For this review, use the dimensioned drawing (mm, ordinates from the lowest corner) and the shaded views. Round coordinates to 2 decimals unless told otherwise and drop trailing zeros. Loops run counter-clockwise (first coordinate to the right, second up) from the corner with the lowest first, then second, coordinate; pieces in that order, holes last.
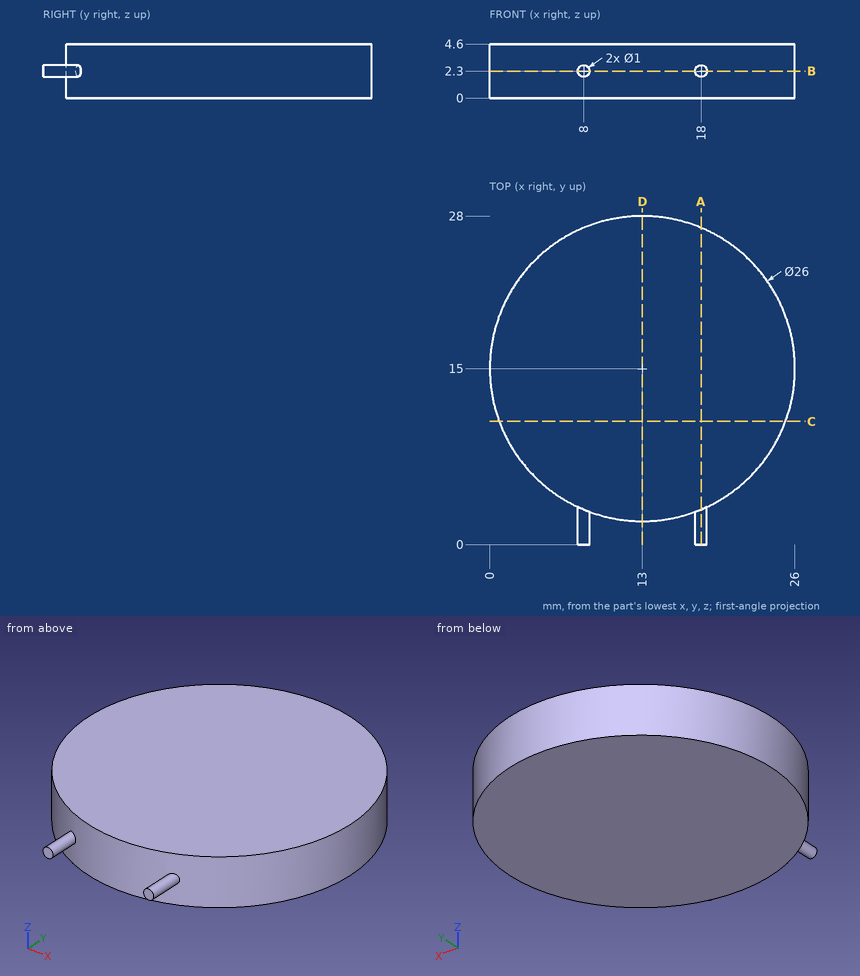
(1) For L1, parallel to Y at x = 2.25, z = 3.25; L2, parallel to Y at x = 15.5, z = 2.3; L3, parallel to X at y = 9.25, z = 2.4, list the stretches that pass through material, from the lowest coordinate up.
(2) Add section A-A (x = 18). Give the boundary of the cut face in (y, z).
(3) Add section D-D (x = 13). Give the boundary of the cut face in (y, z).
(4) Add section B-B (z = 2.3). Give the boundary of the cut face in (x, y).
(5) Add section C-C (y = 10.5). Give the boundary of the cut face in (x, z), plus the area to 3 significant figures.
Outcome:
1. L1: y = 7.69 to 22.31
1. L2: y = 2.24 to 27.76
1. L3: x = 1.34 to 24.66
2. outline: (0, 1.8) - (3, 1.8) - (3, 0) - (27, 0) - (27, 4.6) - (3, 4.6) - (3, 2.8) - (0, 2.8) - close
3. outline: (2, 0) - (28, 0) - (28, 4.6) - (2, 4.6) - close
4. outline: (7.5, 0) - (8.5, 0) - (8.5, 2.8) arc R13 ccw to (17.5, 2.8) - (17.5, 0) - (18.5, 0) - (18.5, 3.22) arc R13 ccw (long way) to (7.5, 3.22) - close
5. outline: (0.8, 0) - (25.2, 0) - (25.2, 4.6) - (0.8, 4.6) - close
5. area: 112 mm2
